Verification items for this drawing (mm, ordinates from the low corner). Round coordinates to 2 decimals unless told otherwise and drop trailing zeros. Order: outer loops, then holes, each group sorted by start corner. A loop starts at its lowest first (then second) coordinate and runs counter-clockwise, first axis right, second up. Notation, with made-up numbers: (-1.5, -25) -> (45.5, -25) arc R27 cw to (45.5, -5) -> close; hole circle Ø1 at (85, 5.25). An arc over 180 degrees is marked (long way). Answer in a Markdown table with one row per item. Add a question column.
1. Sectioned sample at B-B, the plane x = 12.5. Record the boundary of the cut face in (y, z), then the cut area to 3 significant figures.
2. Sectioned sample at A-A, the plane z = 1.55. Record the boundary of the cut face in (x, y).
3. Material ranges on L1, parallel to X at y = 49.5, z = 1.65; L2, parallel to X at y = 56, z = 2.8; L3, parallel to Y at x = 14.5, z = 1.45, recorded low to high. Write a range as from..to.
4. Depth check by flat-ended pin: P1, Ø5, axis at x = 40.5, y = 27.5, coming from the -Z side; P2, Ø0.5, axis at y = 35, z = 3.5, coming from the +X side; P3, Ø1.7, axis at y = 34, z = 3.5, coming from the -X side; P4, Ø0.8, axis at x = 64, z = 3.5, coming from the -Y side. Enter the tip coordinate at first touch or a pass-through.
5. Sectioned sample at D-D, the plane y = 60. Record the boundary of the cut face in (x, z), then the cut area to 3 significant figures.
6. Sectioned sample at C-C, the plane y = 15. Record the boundary of the cut face in (x, z), then the cut area to 3 significant figures.
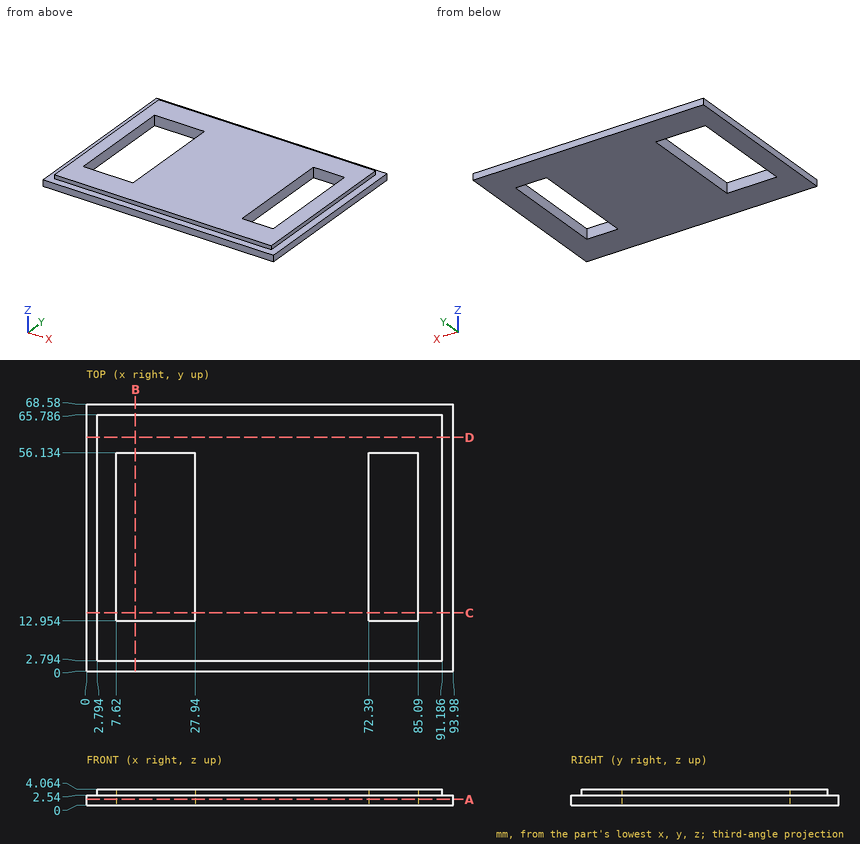
Answer key:
| question | item | result |
|---|---|---|
| 1 | outline | (0, 0) -> (12.95, 0) -> (12.95, 4.06) -> (2.79, 4.06) -> (2.79, 2.54) -> (0, 2.54) -> close; (56.13, 0) -> (68.58, 0) -> (68.58, 2.54) -> (65.79, 2.54) -> (65.79, 4.06) -> (56.13, 4.06) -> close |
| 1 | area | 94.7 mm² |
| 2 | outline | (0, 0) -> (93.98, 0) -> (93.98, 68.58) -> (0, 68.58) -> close; hole (7.62, 12.95) -> (27.94, 12.95) -> (27.94, 56.13) -> (7.62, 56.13) -> close; hole (72.39, 12.95) -> (85.09, 12.95) -> (85.09, 56.13) -> (72.39, 56.13) -> close |
| 3 | L1 | x = 0..7.62, 27.94..72.39, 85.09..93.98 |
| 3 | L2 | x = 2.79..7.62, 27.94..72.39, 85.09..91.19 |
| 3 | L3 | y = 0..12.95, 56.13..68.58 |
| 4 | P1 | stops at z = 0 |
| 4 | P2 | stops at x = 91.19 |
| 4 | P3 | stops at x = 2.79 |
| 4 | P4 | stops at y = 2.79 |
| 5 | outline | (0, 0) -> (93.98, 0) -> (93.98, 2.54) -> (91.19, 2.54) -> (91.19, 4.06) -> (2.79, 4.06) -> (2.79, 2.54) -> (0, 2.54) -> close |
| 5 | area | 373 mm² |
| 6 | outline | (0, 0) -> (7.62, 0) -> (7.62, 4.06) -> (2.79, 4.06) -> (2.79, 2.54) -> (0, 2.54) -> close; (27.94, 0) -> (72.39, 0) -> (72.39, 4.06) -> (27.94, 4.06) -> close; (85.09, 0) -> (93.98, 0) -> (93.98, 2.54) -> (91.19, 2.54) -> (91.19, 4.06) -> (85.09, 4.06) -> close |
| 6 | area | 239 mm² |
